Model file for the job. Use its own axes, mm. A direction names the side the tool comes from. Round coordinates to 2 decimals unless told otherwise and drop trailing zeros. Order: outer loops, then holes, each group sorted by start corner. A loop starts at its lowest first (then second) coordinate and runs counter-clockwise, first axis right, second up. Notation, with made-up numbers: (73.25, 77.25) - (89.25, 77.25) arc R35 cw to (89.25, 110.25) - close; hole circle Ø2 at (-21.5, 87). An arc over 180 degrees is marked (long way). Use one line per item in the form item = value.
from build123d import *

# Parameters (mm, degrees)
SKETCH_R     = 4.1
PAD_DEPTH    = 10
SKETCH001_W  = 3.486151
SKETCH001_H  = 8
PAD001_DEPTH = 1


with BuildPart() as part:
    # Sketch → Pad (new body)
    with BuildSketch(Plane.XY):
        with BuildLine():
            Line((-48.388943, 45.786089), (-48.388943, 33.786089))
            Line((-48.388943, 33.786089), (-52.887429, 17.610197))
            Line((-52.887429, 17.610197), (-50.887429, 17.610197))
            ThreePointArc((-37.388943, 25.561053), (-44.951067, 22.965687), (-50.887429, 17.610197))
            Line((-37.388943, 28.561053), (-37.388943, 25.561053))
            Line((-41.388943, 28.561053), (-37.388943, 28.561053))
            Line((-41.388943, 47.561053), (-41.388943, 28.561053))
            Line((-37.388943, 47.561053), (-41.388943, 47.561053))
            Line((-37.388943, 54.561053), (-37.388943, 47.561053))
            ThreePointArc((-37.388943, 54.561053), (-52.001429, 61.596677), (-48.388943, 45.786089))
        make_face()
        with Locations((-46.388943, 54.561053)):
            Circle(SKETCH_R, mode=Mode.SUBTRACT)
    extrude(amount=PAD_DEPTH)

    # Sketch001 → Pad001 (new body)
    with BuildSketch(Plane.YZ.offset(-37.388943)):
        with Locations((52.817977, 5)):
            Rectangle(SKETCH001_W, SKETCH001_H)
    extrude(amount=PAD001_DEPTH)


solid = part.part
(1) Pin check, flat tips, straight feed: pin 1 (0.5 mm diameter, centred on x = -37, z = 4, fed in from +Y); pin 2 (0.5 mm diameter, centred on x = -37, y = 53.5, fed in from -Z); pin 3 (1.5 mm diameter, centred on y = 27, z = 6.5, fed in from +X). Stop position of each tip, or through.
Report:
pin_1 = 54.56
pin_2 = 1
pin_3 = -37.39
(2) Slice it at D-D on y = 56. Give the cut face in (x, z).
Report:
outline = (-55.27, 0) - (-50.23, 0) - (-50.23, 10) - (-55.27, 10) - close; (-42.55, 0) - (-37.5, 0) - (-37.5, 10) - (-42.55, 10) - close
(3) Tool access for faces 4 (the face through (-48.389, 40, 5)), 5 (the face through (-37, 53, 9)), 6 (the face through (-37.389, 27, 5)), 7 (the face through (-41.389, 38, 5)): list every direction of +Z, -Z, +X, -X, +Y, -Y with a clear straight run to the whole face (end or side of a thin tool).
Report:
face_4 = +Z, -Z, -X
face_5 = +Z, +X, +Y, -Y
face_6 = +Z, -Z, +X, -Y
face_7 = +Z, -Z, +X
(4) Slice it at C-C on x = -49.75. Give the cut face in (y, z), then the cut area to 3 significant figures.
Report:
outline = (19.02, 0) - (28.89, 0) - (28.89, 10) - (19.02, 10) - close; (46.21, 0) - (52.21, 0) - (52.21, 10) - (46.21, 10) - close; (56.91, 0) - (62.91, 0) - (62.91, 10) - (56.91, 10) - close
area = 219 mm2
(5) Slice it at B-B on x = -45. Give the cut face in (y, z).
Report:
outline = (22.94, 0) - (50.7, 0) - (50.7, 10) - (22.94, 10) - close; (58.42, 0) - (63.45, 0) - (63.45, 10) - (58.42, 10) - close
(6) Pull direction Y, two halves, no side cores. Call faces 1 (the face through (-47, 41, 0)), 2 (the face through (-52, 17.61, 5)), 3 (the face through (-39, 47.561, 5)): released by +Y, released by -Y, zero draft, split by the parting line, or undercut.
Report:
face_1 = zero draft
face_2 = released by -Y
face_3 = undercut
(7) Probe probe 1 along X at (y, z) = (37, 5.25); probe 2 along Y at (x, z) = (-46.25, 6.5); probe 3 along X at (y, z) = (57, 3). List the from-to ranges inside material, lowest first. Write a range as [from, to].
Report:
probe_1 = [-48.39, -41.39]
probe_2 = [22.13, 50.46], [58.66, 63.56]
probe_3 = [-55.05, -49.68], [-43.09, -37.73]
(8) Slice it at A-A on z = 5.75. Give the cut face in (x, y).
Report:
outline = (-52.89, 17.61) - (-50.89, 17.61) arc R19.95 cw to (-37.39, 25.56) - (-37.39, 28.56) - (-41.39, 28.56) - (-41.39, 47.56) - (-37.39, 47.56) - (-37.39, 51.07) - (-36.39, 51.07) - (-36.39, 54.56) - (-37.39, 54.56) arc R9 ccw (long way) to (-48.39, 45.79) - (-48.39, 33.79) - close; hole circle Ø8.2 at (-46.39, 54.56)
